Geometry: final body of the model. Coordinates: model frame, mm. Face numbers are marked on the shaded views. Round coordinates to 2 decimals unless told otherwise and drop trailing zeros. Answer as CSV lines item,"result".
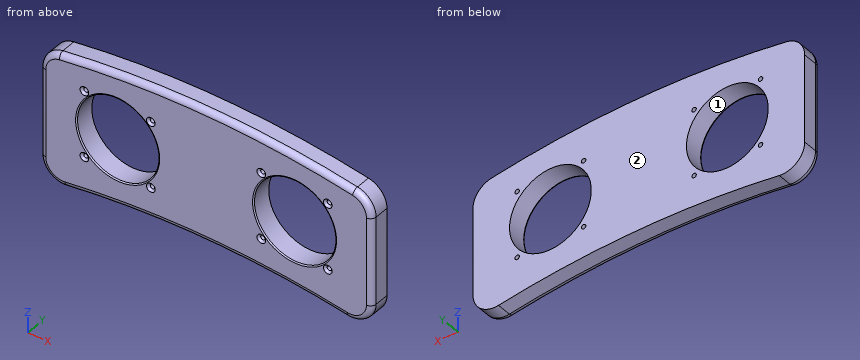
from build123d import *

# Parameters (mm, degrees)
F0_R     = 2
F0_R_2   = 37
F1_DEPTH = 18
F2_R     = 1
F3_R     = 5
F4_SIZE  = 1.9


with BuildPart() as f1:
    # F0 (on Front) → F1 (new body)
    with BuildSketch(Plane.XZ):
        with BuildLine():
            ThreePointArc((-133.204654, 99.258737), (-145.233074, 92.476837), (-150, 79.517151))
            Line((-150, 79.517151), (-150, 0.01569))
            ThreePointArc((-150, 0.01569), (-143.017649, -15.16788), (-126.945919, -19.74975))
            ThreePointArc((-126.945919, -19.74975), (0, -10), (126.945919, -19.74975))
            ThreePointArc((126.945919, -19.74975), (143.017649, -15.16788), (150, 0.01569))
            Line((150, 0.01569), (150, 79.517151))
            ThreePointArc((150, 79.517151), (145.233074, 92.476837), (133.204654, 99.258737))
            ThreePointArc((133.204654, 99.258737), (0, 110), (-133.204654, 99.258737))
        make_face()
        with Locations((-110.052038, 16.089709)):
            Circle(F0_R, mode=Mode.SUBTRACT)
        with Locations((-49.947962, 16.089709)):
            Circle(F0_R, mode=Mode.SUBTRACT)
        with Locations((49.947962, 16.089709)):
            Circle(F0_R, mode=Mode.SUBTRACT)
        with Locations((110.052038, 16.089709)):
            Circle(F0_R, mode=Mode.SUBTRACT)
        with Locations((-80, 46.141747)):
            Circle(F0_R_2, mode=Mode.SUBTRACT)
        with Locations((-110.052038, 76.193785)):
            Circle(F0_R, mode=Mode.SUBTRACT)
        with Locations((-49.947962, 76.193785)):
            Circle(F0_R, mode=Mode.SUBTRACT)
        with Locations((49.947962, 76.193785)):
            Circle(F0_R, mode=Mode.SUBTRACT)
        with Locations((80, 46.141747)):
            Circle(F0_R_2, mode=Mode.SUBTRACT)
        with Locations((110.052038, 76.193785)):
            Circle(F0_R, mode=Mode.SUBTRACT)
    extrude(amount=-F1_DEPTH)

    # F2
    f2_edges = [f1.edges().sort_by_distance(p)[0] for p in [
        (-117, 0, 46.141747),
        (43, 0, 46.141747),
    ]]
    fillet(f2_edges, radius=F2_R)

    # F3
    f3_edges = [f1.edges().sort_by_distance(p)[0] for p in [
        (0, 0, 110),
        (145.233074, 0, 92.476837),
        (150, 0, 39.766421),
        (143.017649, 0, -15.16788),
        (0, 0, -10),
        (-143.017649, 0, -15.16788),
        (-150, 0, 39.766421),
        (-145.233074, 0, 92.476837),
    ]]
    fillet(f3_edges, radius=F3_R)

    # F4
    f4_edges = [f1.edges().sort_by_distance(p)[0] for p in [
        (-112.052038, 0, 76.193785),
        (-51.947962, 0, 76.193785),
        (-112.052038, 0, 16.089709),
        (-51.947962, 0, 16.089709),
        (47.947962, 0, 16.089709),
        (47.947962, 0, 76.193785),
        (108.052038, 0, 16.089709),
        (108.052038, 0, 76.193785),
    ]]
    chamfer(f4_edges, length=F4_SIZE)


solid = f1.part
(1) Section A-A (y = 8.25). Give the number of separate pieces and of enclosed holes in the cut face, and give its area (3 significant figures).
Findings below:
separate pieces,"1"
enclosed holes,"10"
area,"26,900 mm2"
(2) Pin query (flat end, axial travel): P1, Ø5, axis at x = -49.95, z = 16.09, coming from the -Y side; P2, Ø6.5, axis at x = 110.05, z = 76.19, coming from the -Y side; P3, Ø4.5, axis at x = -110.05, z = 76.19, coming from the -Y side. Return the tip coordinate at first contact, or that it passes through.
Findings below:
P1,"y = 1.4"
P2,"y = 0.65"
P3,"y = 1.65"
(3) Draft query along Z for the marked faces 1 and 2. Return one class per face: pulls with the +Z half, pulls with the -Z half, needs draft (parallel to the pull), parting line crosses it, or undercut.
Findings below:
face 1,"undercut"
face 2,"needs draft"
(4) Material intervals for line 1 along X through (y, z) = (9.25, 42.5); line 2 along X through (y, z) = (4.25, 35.5); line 3 along Z through (x, y) = (-96, 7.5), sorted ascending.
Findings below:
line 1,"-150 to -116.82, -43.18 to 43.18, 116.82 to 150"
line 2,"-149.94 to -115.44, -44.56 to 44.56, 115.44 to 149.94"
line 3,"-15.56 to 12.78, 79.5 to 104.44"
